CAD build for the part. Positions are in the model's coordinates, mm. Round coordinates to 2 decimals unless told otherwise and drop trailing zeros. Write each loop counter-clockwise with the first axis right and the second up, starting at its lowest first coordinate (ties: lowest second). Pieces come first, ordered by that corner, then holes. Notation, with made-up numbers: (58, -40) - (88, -40) arc R10 ccw to (88, -23) - close; hole circle Ø3 at (-4, 81). An arc over 180 degrees is marked (long way). Use one line per item in the form item = value. Start each with the question number.
Item 1: Band-saw the part on C-C, the plane x = 38.1. List the corners of the cut face in (y, z).
Item 2: Band-saw the part on A-A, the plane y = 25.4. List the corners of the cut face in (x, z).
Item 3: Drill centre lines: L1, parallel to Y at x = 57, z = 3.2; L2, parallel to Y at x = 67, z = 2.9; L3, parallel to X at y = 12, z = 3.15. Where is each one in solid material? Low to high.
Item 4: Pull direction Y, two halves, no side cores. Call faces 1 (the cylindrical face through (68.6, 42.9, 2.3)), 2 (the flat face through (38, 50.8, 2)), 3 (the flat face through (20.6, 31.4, 4.572)): +Y half, -Y half, draft (parallel to the pull), parting line (faces both ways), or undercut.
Item 5: Band-saw the part on B-B, the plane x = 19.05. List the corners of the cut face in (y, z), and give its area (3 significant figures).
Item 6: Band-saw the part on D-D, the plane z = 2.65. Give the number of separate pieces and of enclosed holes in the cut face, and give its area (3 significant figures).
from build123d import *

# Parameters (mm, degrees)
SKETCH1_W               = 76.2
SKETCH1_H               = 50.8
BOSS_EXTRUDE1_DEPTH     = 4.572
CAVITY5_OUTLINE_R       = 18.161
CAVITY5_OUTLINE_R_2     = 0.889
CAVITY5_DEPTH           = 4.572
SKETCH3_R               = 1.5875
CUT_EXTRUDE1_DEPTH      = 92.695055396
MIRROR2_COPY_1_SKETCH_R = 1.5875
MIRROR2_COPY_1_DEPTH    = 92.695055396
SKETCH4_R               = 1.5875
CUT_EXTRUDE2_DEPTH      = 92.695055396


# Read off the part's stored shape, not the designer's step: Cavity5
with BuildPart() as part:
    # Sketch1 → Boss-Extrude1 (new body)
    with BuildSketch(Plane.XY):
        with Locations((38.1, 25.4)):
            Rectangle(SKETCH1_W, SKETCH1_H)
    extrude(amount=BOSS_EXTRUDE1_DEPTH)

    # Cavity5 outline → Cavity5 (cut)
    with BuildSketch(Plane.XY):
        with Locations((38.1, 25.4)):
            Circle(CAVITY5_OUTLINE_R)
        with Locations((16.188175065, 25.4)):
            Circle(CAVITY5_OUTLINE_R_2)
        with Locations((60.011824935, 25.4)):
            Circle(CAVITY5_OUTLINE_R_2)
    extrude(amount=CAVITY5_DEPTH, mode=Mode.SUBTRACT)

    # Sketch3 → Cut-Extrude1 (cut, through all)
    with BuildSketch(Plane(origin=(0, 0, 0), x_dir=(-1, 0, 0), z_dir=(0, 0, -1))):
        with Locations((-68.2625, 44.45)):
            Circle(SKETCH3_R)
    cut_extrude1 = extrude(amount=-CUT_EXTRUDE1_DEPTH, mode=Mode.SUBTRACT)

    # Mirror1: Cut-Extrude1 across plane
    add(cut_extrude1.mirror(Plane(origin=(38.1, 0, 0), x_dir=(0, 0, 1), z_dir=(1, 0, 0))), mode=Mode.SUBTRACT)

    # Mirror2: Cut-Extrude1 across plane
    add(cut_extrude1.mirror(Plane.ZX.offset(25.4)), mode=Mode.SUBTRACT)

    # Mirror2 copy 1 sketch → Mirror2 copy 1 (cut, through all)
    with BuildSketch(Plane(origin=(76.2, 50.8, 0), x_dir=(1, 0, 0), z_dir=(0, 0, -1))):
        with Locations((-68.2625, 44.45)):
            Circle(MIRROR2_COPY_1_SKETCH_R)
    extrude(amount=-MIRROR2_COPY_1_DEPTH, mode=Mode.SUBTRACT)

    # Sketch4 → Cut-Extrude2 (cut, through all)
    with BuildSketch(Plane(origin=(0, 0, 0), x_dir=(-1, 0, 0), z_dir=(0, 0, -1))):
        with Locations((-19.05, 44.45)):
            Circle(SKETCH4_R)
        with Locations((-57.15, 44.45)):
            Circle(SKETCH4_R)
        with Locations((-57.15, 6.35)):
            Circle(SKETCH4_R)
        with Locations((-19.05, 6.35)):
            Circle(SKETCH4_R)
    extrude(amount=-CUT_EXTRUDE2_DEPTH, mode=Mode.SUBTRACT)


solid = part.part
Determined:
q1.outline = (0, 0) - (7.24, 0) - (7.24, 4.57) - (0, 4.57) - close; (43.56, 0) - (50.8, 0) - (50.8, 4.57) - (43.56, 4.57) - close
q2.outline = (0, 0) - (15.3, 0) - (15.3, 4.57) - (0, 4.57) - close; (17.08, 0) - (19.94, 0) - (19.94, 4.57) - (17.08, 4.57) - close; (56.26, 0) - (59.12, 0) - (59.12, 4.57) - (56.26, 4.57) - close; (60.9, 0) - (76.2, 0) - (76.2, 4.57) - (60.9, 4.57) - close
q3.L1 = 0 to 4.77, 7.93 to 42.87, 46.03 to 50.8
q3.L2 = 0 to 5.39, 7.31 to 43.49, 45.41 to 50.8
q3.L3 = 0 to 25.84, 50.36 to 76.2
q4.face_1 = undercut
q4.face_2 = +Y half
q4.face_3 = draft
q5.outline = (0, 0) - (4.76, 0) - (4.76, 4.57) - (0, 4.57) - close; (7.94, 0) - (42.86, 0) - (42.86, 4.57) - (7.94, 4.57) - close; (46.04, 0) - (50.8, 0) - (50.8, 4.57) - (46.04, 4.57) - close
q5.area = 203 mm²
q6.separate_pieces = 1
q6.enclosed_holes = 11
q6.area = 2,770 mm²
